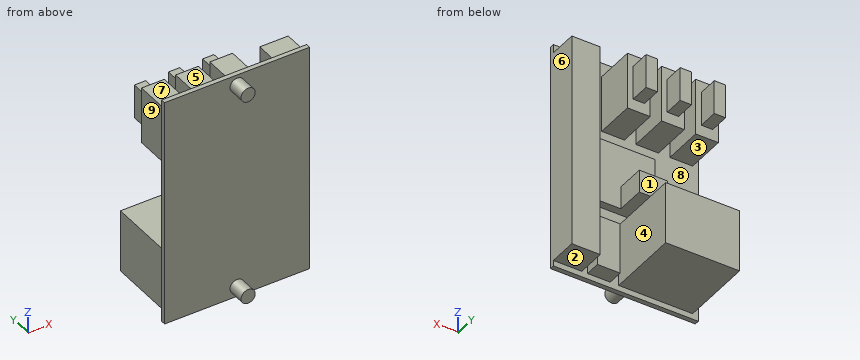
from build123d import *

# Parameters (mm, degrees)
SK_P01_STANDOFF_R                  = 2.5
P01_STANDOFF_DEPTH                 = 6
SK_P02_STANDOFF_R                  = 2.5
P02_STANDOFF_DEPTH                 = 6
P03_PERMAPROTOHALFSIZEBOARD_START  = 6
SK_P03_PERMAPROTOHALFSIZEBOARD_W   = 51
SK_P03_PERMAPROTOHALFSIZEBOARD_H   = 81
P03_PERMAPROTOHALFSIZEBOARD_DEPTH  = 1.6
P04_K1RELAYCB1AFP12V_START         = 7.6
SK_P04_K1RELAYCB1AFP12V_W          = 26
SK_P04_K1RELAYCB1AFP12V_H          = 22
P04_K1RELAYCB1AFP12V_DEPTH         = 25.5
P05_R1D3D4K1COIL_START             = 7.6
SK_P05_R1D3D4K1COIL_W              = 8
SK_P05_R1D3D4K1COIL_H              = 18
P05_R1D3D4K1COIL_DEPTH             = 5.4
P06_INA2601MOTOR_START             = 7.6
SK_P06_INA2601MOTOR_W              = 22.9
SK_P06_INA2601MOTOR_H              = 22.8
P06_INA2601MOTOR_DEPTH             = 2.7
P07_INA260TERMINALBLOCK_START      = 10.3
SK_P07_INA260TERMINALBLOCK_W       = 10
SK_P07_INA260TERMINALBLOCK_H       = 8
P07_INA260TERMINALBLOCK_DEPTH      = 10
P08_F1HOLDER30APCBBLADE_START      = 7.6
SK_P08_F1HOLDER30APCBBLADE_W       = 8
SK_P08_F1HOLDER30APCBBLADE_H       = 20
P08_F1HOLDER30APCBBLADE_DEPTH      = 14
P09_F115AFUSE_START                = 21.6
SK_P09_F115AFUSE_W                 = 4
SK_P09_F115AFUSE_H                 = 12
P09_F115AFUSE_DEPTH                = 7
P10_F3HOLDER_START                 = 7.6
SK_P10_F3HOLDER_W                  = 8
SK_P10_F3HOLDER_H                  = 20
P10_F3HOLDER_DEPTH                 = 14
P11_F33AFUSE_START                 = 21.6
SK_P11_F33AFUSE_W                  = 4
SK_P11_F33AFUSE_H                  = 12
P11_F33AFUSE_DEPTH                 = 7
P12_F4HOLDER_START                 = 7.6
SK_P12_F4HOLDER_W                  = 8
SK_P12_F4HOLDER_H                  = 20
P12_F4HOLDER_DEPTH                 = 14
P13_F43AFUSE_START                 = 21.6
SK_P13_F43AFUSE_W                  = 4
SK_P13_F43AFUSE_H                  = 12
P13_F43AFUSE_DEPTH                 = 7
P14_TERMINALBLOCKSTB1TB4WIRE_START = 7.6
SK_P14_TERMINALBLOCKSTB1TB4WIRE_W  = 10
SK_P14_TERMINALBLOCKSTB1TB4WIRE_H  = 76
P14_TERMINALBLOCKSTB1TB4WIRE_DEPTH = 10


with BuildPart() as part:
    # SK_P01_Standoff → P01_Standoff (new body)
    with BuildSketch(Plane(origin=(0, 0, 0), x_dir=(1, 0, 0), z_dir=(0, 1, 0))):
        with Locations(Location((0, 36.85, 0), (0, 0, 270))):
            Circle(SK_P01_STANDOFF_R)
    extrude(amount=P01_STANDOFF_DEPTH)



with BuildPart() as body_2:
    # SK_P02_Standoff → P02_Standoff (new body)
    with BuildSketch(Plane(origin=(0, 0, 0), x_dir=(1, 0, 0), z_dir=(0, 1, 0))):
        with Locations(Location((0, -36.85, 0), (0, 0, 270))):
            Circle(SK_P02_STANDOFF_R)
    extrude(amount=P02_STANDOFF_DEPTH)


with BuildPart() as part_1:
    add(part.part)

    add(body_2.part)  # P03_PermaProtohalfsizeboard merges body 2
    # SK_P03_PermaProtohalfsizeboard → P03_PermaProtohalfsizeboard (add)
    with BuildSketch(Plane(origin=(0, 0, 0), x_dir=(1, 0, 0), z_dir=(0, 1, 0)).offset(P03_PERMAPROTOHALFSIZEBOARD_START)):
        Rectangle(SK_P03_PERMAPROTOHALFSIZEBOARD_W, SK_P03_PERMAPROTOHALFSIZEBOARD_H)
    extrude(amount=P03_PERMAPROTOHALFSIZEBOARD_DEPTH)

    # SK_P04_K1relayCB1aFP12V → P04_K1relayCB1aFP12V (add)
    with BuildSketch(Plane(origin=(0, 0, 0), x_dir=(1, 0, 0), z_dir=(0, 1, 0)).offset(P04_K1RELAYCB1AFP12V_START)):
        with Locations((-10.5, 27.5)):
            Rectangle(SK_P04_K1RELAYCB1AFP12V_W, SK_P04_K1RELAYCB1AFP12V_H)
    extrude(amount=P04_K1RELAYCB1AFP12V_DEPTH)

    # SK_P05_R1D3D4K1coil → P05_R1D3D4K1coil (add)
    with BuildSketch(Plane(origin=(0, 0, 0), x_dir=(1, 0, 0), z_dir=(0, 1, 0)).offset(P05_R1D3D4K1COIL_START)):
        with Locations((9.5, 29.5)):
            Rectangle(SK_P05_R1D3D4K1COIL_W, SK_P05_R1D3D4K1COIL_H)
    extrude(amount=P05_R1D3D4K1COIL_DEPTH)

    # SK_P06_INA2601motor → P06_INA2601motor (add)
    with BuildSketch(Plane(origin=(0, 0, 0), x_dir=(1, 0, 0), z_dir=(0, 1, 0)).offset(P06_INA2601MOTOR_START)):
        with Locations((2.95, 1.1)):
            Rectangle(SK_P06_INA2601MOTOR_W, SK_P06_INA2601MOTOR_H)
    extrude(amount=P06_INA2601MOTOR_DEPTH)

    # SK_P07_INA260terminalblock → P07_INA260terminalblock (add)
    with BuildSketch(Plane(origin=(0, 0, 0), x_dir=(1, 0, 0), z_dir=(0, 1, 0)).offset(P07_INA260TERMINALBLOCK_START)):
        with Locations((-1.5, 8.5)):
            Rectangle(SK_P07_INA260TERMINALBLOCK_W, SK_P07_INA260TERMINALBLOCK_H)
    extrude(amount=P07_INA260TERMINALBLOCK_DEPTH)

    # SK_P08_F1holder30APCBblade → P08_F1holder30APCBblade (add)
    with BuildSketch(Plane(origin=(0, 0, 0), x_dir=(1, 0, 0), z_dir=(0, 1, 0)).offset(P08_F1HOLDER30APCBBLADE_START)):
        with Locations((-19.5, -25.5)):
            Rectangle(SK_P08_F1HOLDER30APCBBLADE_W, SK_P08_F1HOLDER30APCBBLADE_H)
    extrude(amount=P08_F1HOLDER30APCBBLADE_DEPTH)

    # SK_P09_F115Afuse → P09_F115Afuse (add)
    with BuildSketch(Plane(origin=(0, 0, 0), x_dir=(1, 0, 0), z_dir=(0, 1, 0)).offset(P09_F115AFUSE_START)):
        with Locations((-19.5, -25.5)):
            Rectangle(SK_P09_F115AFUSE_W, SK_P09_F115AFUSE_H)
    extrude(amount=P09_F115AFUSE_DEPTH)

    # SK_P10_F3holder → P10_F3holder (add)
    with BuildSketch(Plane(origin=(0, 0, 0), x_dir=(1, 0, 0), z_dir=(0, 1, 0)).offset(P10_F3HOLDER_START)):
        with Locations((-7.5, -25.5)):
            Rectangle(SK_P10_F3HOLDER_W, SK_P10_F3HOLDER_H)
    extrude(amount=P10_F3HOLDER_DEPTH)

    # SK_P11_F33Afuse → P11_F33Afuse (add)
    with BuildSketch(Plane(origin=(0, 0, 0), x_dir=(1, 0, 0), z_dir=(0, 1, 0)).offset(P11_F33AFUSE_START)):
        with Locations((-7.5, -25.5)):
            Rectangle(SK_P11_F33AFUSE_W, SK_P11_F33AFUSE_H)
    extrude(amount=P11_F33AFUSE_DEPTH)

    # SK_P12_F4holder → P12_F4holder (add)
    with BuildSketch(Plane(origin=(0, 0, 0), x_dir=(1, 0, 0), z_dir=(0, 1, 0)).offset(P12_F4HOLDER_START)):
        with Locations((4.5, -25.5)):
            Rectangle(SK_P12_F4HOLDER_W, SK_P12_F4HOLDER_H)
    extrude(amount=P12_F4HOLDER_DEPTH)

    # SK_P13_F43Afuse → P13_F43Afuse (add)
    with BuildSketch(Plane(origin=(0, 0, 0), x_dir=(1, 0, 0), z_dir=(0, 1, 0)).offset(P13_F43AFUSE_START)):
        with Locations((4.5, -25.5)):
            Rectangle(SK_P13_F43AFUSE_W, SK_P13_F43AFUSE_H)
    extrude(amount=P13_F43AFUSE_DEPTH)

    # SK_P14_TerminalblocksTB1TB4wire → P14_TerminalblocksTB1TB4wire (add)
    with BuildSketch(Plane(origin=(0, 0, 0), x_dir=(1, 0, 0), z_dir=(0, 1, 0)).offset(P14_TERMINALBLOCKSTB1TB4WIRE_START)):
        with Locations((20.5, 0.5)):
            Rectangle(SK_P14_TERMINALBLOCKSTB1TB4WIRE_W, SK_P14_TERMINALBLOCKSTB1TB4WIRE_H)
    extrude(amount=P14_TERMINALBLOCKSTB1TB4WIRE_DEPTH)


solid = part_1.part
Read the model definition and answer for the solid it produces. Units are mm, in the model's axes. Face numbers are marked on the shaded views. A direction names the side the tool comes from. Round coordinates to 2 decimals unless told otherwise and drop trailing zeros. Write each loop counter-clockwise with the first axis right and the second up, starting at its lowest first coordinate (ties: lowest second). Pieces come first, ordered by that corner, then holes.
1. The part is cut by section C-C, the plane x = 19.5. Determine the outline of the cut face in (y, z).
2. Straight lines are drawn through the part: L1, parallel to X at y = 26, z = 24; L2, parallel to Z at x = 13, y = 8; L3, parallel to X at y = 17, z = -8. For each, find the intervals that lie inside material, in ascending order.
3. The part is cut by section B-B, the plane z = 1.5. Determine the outline of the cut face in (x, y).
4. Which of the six approach directions +Z, -Z, +X, -X, +Y, -Y give full straight-line access (tool end or side, diameter ignored) to the marked faces 1, 2, 3, 4 and 5?
5. Determine the mould class of the marked faces 6, 7, 8 and 9 for opening direction X: pulls with the +X half, pulls with the -X half, needs draft (parallel to the pull), parting line crosses it, or undercut.
6. The part is cut by section A-A, the plane y = 23. Determine the outline of the cut face in (x, z), then the cut area to 3 significant figures.
7. Given pin 1 Ø8 at (x, z) = (-13, 4.5) entering from -Y; pin 2 Ø10 at (x, z) = (-7.5, -8) entering from +Y; pin 3 Ø5.5 at (y, z) = (24, 25.5) entering from +X; pin 4 Ø5 at (y, z) = (26, -13) entering from +X, each flat-ended and moving along its own axis, determine where each tip first touches the part or whether it passes through.
Values:
1. outline: (6, -40.5) - (7.6, -40.5) - (7.6, -38.5) - (17.6, -38.5) - (17.6, 37.5) - (7.6, 37.5) - (7.6, 40.5) - (6, 40.5) - close
2. L1: x = -21.5 to -17.5, -9.5 to -5.5, 2.5 to 6.5
2. L2: z = -38.5 to -20.5, -12.5 to 10.3
2. L3: x = -6.5 to 3.5, 15.5 to 25.5
3. outline: (-25.5, 6) - (25.5, 6) - (25.5, 17.6) - (15.5, 17.6) - (15.5, 7.6) - (14.4, 7.6) - (14.4, 10.3) - (-8.5, 10.3) - (-8.5, 7.6) - (-25.5, 7.6) - close
4. face 1: +X, -X, +Y
4. face 2: -Z, +X, -X, +Y
4. face 3: -X, +Y
4. face 4: -Z, +Y
4. face 5: +Z, -X, +Y
5. face 6: pulls with the +X half
5. face 7: needs draft
5. face 8: undercut
5. face 9: pulls with the -X half
6. outline: (-23.5, -38.5) - (2.5, -38.5) - (2.5, -16.5) - (-23.5, -16.5) - close; (-21.5, 19.5) - (-17.5, 19.5) - (-17.5, 31.5) - (-21.5, 31.5) - close; (-9.5, 19.5) - (-5.5, 19.5) - (-5.5, 31.5) - (-9.5, 31.5) - close; (2.5, 19.5) - (6.5, 19.5) - (6.5, 31.5) - (2.5, 31.5) - close
6. area: 716 mm2
7. pin 1: stops at y = 6
7. pin 2: stops at y = 20.3
7. pin 3: stops at x = 8.5
7. pin 4: passes through
